Input: part model. Units: mm. Frame: model coordinates. Face numbers are marked on the shaded views. A direction names the side the tool comes from. Give positions to 0.01 mm unless a question says otherwise; leave off trailing zeros. Order: outer loops, then holes, each group sorted by start corner. A loop starts at its lowest first (then second) coordinate and runs counter-clockwise, first axis right, second up. Notation, with made-up numbers: (-8, -10.75) - (17, -10.75) arc R6 ccw to (17, -3.75) - close; hole circle Ø2 at (76, 61.25). An arc over 180 degrees is marked (long way). Answer in a Markdown table with one row per item. Add a question column.
from build123d import *

# Parameters (mm, degrees)
BOSS_EXTRUDE1_DEPTH = 800
SHELL1_T            = -1


with BuildPart() as part:
    # Sketch1 → Boss-Extrude1 (new body)
    with BuildSketch(Plane.XY):
        Polygon((-978.315410822, 0), (-548.315410822, 0), (-288.507789686, 150), (-1238.123031957, 150), align=None)
    extrude(amount=BOSS_EXTRUDE1_DEPTH)

    # Shell1
    shell1_openings = [part.faces().sort_by_distance(p)[0] for p in [
        (-763.315410822, 150, 400),
    ]]
    offset(amount=SHELL1_T, openings=shell1_openings, kind=Kind.INTERSECTION)


solid = part.part
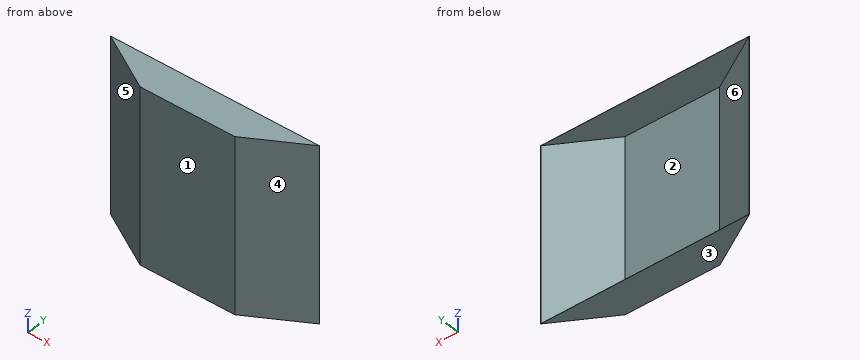
Q1. Section B-B, the plane y = 44.5. Return loops of the section in (x, z).
Q2. Section A-A, the plane x = -852.5. Return loops of the section in (y, z).
Q3. Section C-C, the plane z = 404.5. Return loops of the section in (x, y).
Q4. Line query: probe 1 along Z at (x, y) = (-766.5, 84.5); probe 2 along X at (y, z) = (44, 150); probe 3 along X at (y, z) = (106, 338.5). Output: solid intervals per line, ascending.
Q5. Section D-D, the plane y = 135. Return loops of the section in (x, z).
Q6. Pull-direction query (X, two-part tool) for the marked faces 3, 4, 5 and 6; classes: +X half, -X half, draft (parallel to the pull), parting line (faces both ways), or undercut.
Q7. Access query for the marked faces 1 and 2. Directions: +Z, -Z, +X, -X, +Y, -Y. A direction counts if a zero-diameter tool reaches every point of the face in a straight line with its end or side. Return the directions, or none.
Q8. Contact query for flat-ended pins moving along their axis: P1, Ø4, axis at x = -620, z = 701.5, coming from the +Y side; P2, Ø10, axis at x = -1035.5, z = 455.5, coming from the +Y side; P3, Ø6, axis at y = 78, z = 695, coming from the -X side; P4, Ø3, axis at x = -973, y = 110, coming from the -Z side. Output: stop coordinate, or through.
Computed:
| question | item | result |
|---|---|---|
| 1 | outline | (-1055.39, 0) - (-471.24, 0) - (-471.24, 800) - (-1055.39, 800) - close; hole (-1053.39, 1) - (-473.24, 1) - (-473.24, 799) - (-1053.39, 799) - close |
| 2 | outline | (0, 0) - (150, 0) - (150, 1) - (1, 1) - (1, 799) - (150, 799) - (150, 800) - (0, 800) - close |
| 3 | outline | (-1238.12, 150) - (-978.32, 0) - (-548.32, 0) - (-288.51, 150) - (-290.51, 150) - (-548.58, 1) - (-978.05, 1) - (-1236.12, 150) - close |
| 4 | probe 1 | z = 0 to 1, 799 to 800 |
| 4 | probe 2 | x = -1054.53 to -1052.53, -474.11 to -472.11 |
| 4 | probe 3 | x = -1161.91 to -1159.91, -366.72 to -364.72 |
| 5 | outline | (-1212.14, 0) - (-314.49, 0) - (-314.49, 800) - (-1212.14, 800) - close; hole (-1210.14, 1) - (-316.49, 1) - (-316.49, 799) - (-1210.14, 799) - close |
| 6 | face 3 | draft |
| 6 | face 4 | +X half |
| 6 | face 5 | -X half |
| 6 | face 6 | undercut |
| 7 | face 1 | +Z, -Z, +X, -X, -Y |
| 7 | face 2 | +Y |
| 8 | P1 | stops at y = 1 |
| 8 | P2 | stops at y = 37.06 |
| 8 | P3 | stops at x = -1118.61 |
| 8 | P4 | stops at z = 0 |
